The model under review builds one solid part; all positions refer to its coordinate system, in mm. A direction names the side the tool comes from. Give positions to 0.01 mm unless a question says otherwise; leave off trailing zeros. Loops run counter-clockwise (first coordinate to the right, second up) from the corner with the lowest first, then second, coordinate; pieces in that order, holes last. Notation, with made-up numbers: M -2.5,15 L 46.5,15 A26 ccw 46.5,45 Z; hole C -14.5,67 d2. An arc over 180 degrees is marked long. Return JSON: item names as keys, results as strings. Group by question number.
```python
from build123d import *

# Parameters (mm, degrees)
SKETCH1_W            = 58.42
SKETCH1_H            = 27.94
BOSS_EXTRUDE1_DEPTH  = 27.686
SKETCH2_W            = 0.889
SKETCH2_H            = 8.636
SKETCH2_W_2          = 0.254
SKETCH2_H_2          = 1.905
BOSS_EXTRUDE3_DEPTH  = 27.686
CUT_EXTRUDE1_DEPTH   = 27.305
CUT_EXTRUDE3_DEPTH   = 50.528860243
SKETCH6_W            = 0.508
SKETCH6_H            = 1.778
SKETCH6_W_2          = 0.8128
SKETCH6_H_2          = 1.27
SKETCH6_H_3          = 8.636
BOSS_EXTRUDE4_DEPTH  = 27.686
SKETCH7_W            = 1.3462
SKETCH7_H            = 6.223
CUT_EXTRUDE4_DEPTH   = 25.4
SKETCH8_R            = 1.651
CUT_EXTRUDE5_DEPTH   = 44.216030588
SKETCH9_R            = 2.54
CUT_EXTRUDE6_DEPTH   = 25.4
BOSS_EXTRUDE5_DEPTH  = 1.016
MIRROR3_COPY_1_DEPTH = 1.016


with BuildPart() as part:
    # Sketch1 → Boss-Extrude1 (new body)
    with BuildSketch(Plane.XY):
        Rectangle(SKETCH1_W, SKETCH1_H)
    extrude(amount=BOSS_EXTRUDE1_DEPTH)

    # Sketch2 → Boss-Extrude3 (add)
    with BuildSketch(Plane.XY.offset(27.686)):
        with Locations((-29.6545, 0)):
            Rectangle(SKETCH2_W, SKETCH2_H)
        with Locations((-29.337, 13.0175)):
            Rectangle(SKETCH2_W_2, SKETCH2_H_2)
        with Locations((-29.337, -13.0175)):
            Rectangle(SKETCH2_W_2, SKETCH2_H_2)
        with Locations((29.337, -13.0175)):
            Rectangle(SKETCH2_W_2, SKETCH2_H_2)
        with Locations((29.337, 13.0175)):
            Rectangle(SKETCH2_W_2, SKETCH2_H_2)
        with Locations((29.6545, 0)):
            Rectangle(SKETCH2_W, SKETCH2_H)
    extrude(amount=-BOSS_EXTRUDE3_DEPTH)

    # Sketch4 → Cut-Extrude1 (cut, symmetric)
    with BuildSketch(Plane(origin=(0, 0, 0), x_dir=(0, 0, -1), z_dir=(1, 0, 0))):
        with BuildLine():
            Line((-15.5575, 13.0175), (-27.686, 13.0175))
            Line((-27.686, 13.0175), (-27.686, -13.0175))
            Line((-27.686, -13.0175), (-15.5575, -13.0175))
            ThreePointArc((-15.5575, -13.0175), (-2.54, 0), (-15.5575, 13.0175))
        make_face()
    extrude(amount=CUT_EXTRUDE1_DEPTH, both=True, mode=Mode.SUBTRACT)

    # Sketch5 → Cut-Extrude3 (cut, through all)
    with BuildSketch(Plane.XZ.offset(13.97)):
        with BuildLine():
            Line((-27.305, 27.686), (-27.305, 18.669))
            Line((-27.305, 18.669), (-23.037688998, 18.669))
            ThreePointArc((-23.037688998, 18.669), (-21.720466793, 18.382866674), (-20.640662648, 17.576039787))
            Line((-20.640662648, 17.576039787), (-15.589726503, 11.760960213))
            ThreePointArc((-15.589726503, 11.760960213), (-14.509922358, 10.954133326), (-13.192700152, 10.668))
            Line((-13.192700152, 10.668), (-10.541, 10.668))
            ThreePointArc((-10.541, 10.668), (-8.29593597, 9.73806403), (-7.366, 7.493))
            Line((-7.366, 7.493), (-7.366, 5.588))
            Line((-7.366, 5.588), (7.366, 5.588))
            Line((7.366, 5.588), (7.366, 7.493))
            ThreePointArc((7.366, 7.493), (8.29593597, 9.73806403), (10.541, 10.668))
            Line((10.541, 10.668), (13.192700152, 10.668))
            ThreePointArc((13.192700152, 10.668), (14.509922358, 10.954133326), (15.589726503, 11.760960213))
            Line((15.589726503, 11.760960213), (20.640662648, 17.576039787))
            ThreePointArc((20.640662648, 17.576039787), (21.720466793, 18.382866674), (23.037688998, 18.669))
            Line((23.037688998, 18.669), (27.305, 18.669))
            Line((27.305, 18.669), (27.305, 27.686))
            Line((27.305, 27.686), (-27.305, 27.686))
        make_face()
    extrude(amount=-CUT_EXTRUDE3_DEPTH, mode=Mode.SUBTRACT)

    # Sketch6 → Boss-Extrude4 (add)
    with BuildSketch(Plane.XY.offset(27.686)):
        with Locations((-27.051, 13.081)):
            Rectangle(SKETCH6_W, SKETCH6_H)
        with Locations((-26.8986, 7.747)):
            Rectangle(SKETCH6_W_2, SKETCH6_H_2)
        with Locations((-26.8986, 0)):
            Rectangle(SKETCH6_W_2, SKETCH6_H_3)
        with Locations((-26.8986, -7.747)):
            Rectangle(SKETCH6_W_2, SKETCH6_H_2)
        with Locations((-27.051, -13.081)):
            Rectangle(SKETCH6_W, SKETCH6_H)
        with Locations((27.051, -13.081)):
            Rectangle(SKETCH6_W, SKETCH6_H)
        with Locations((26.8986, -7.747)):
            Rectangle(SKETCH6_W_2, SKETCH6_H_2)
        with Locations((26.8986, 0)):
            Rectangle(SKETCH6_W_2, SKETCH6_H_3)
        with Locations((26.8986, 7.747)):
            Rectangle(SKETCH6_W_2, SKETCH6_H_2)
        with Locations((27.051, 13.081)):
            Rectangle(SKETCH6_W, SKETCH6_H)
    extrude(amount=-BOSS_EXTRUDE4_DEPTH)

    # Sketch7 → Cut-Extrude4 (cut)
    with BuildSketch(Plane.XY.offset(27.686)):
        with Locations((-27.1653, 0)):
            Rectangle(SKETCH7_W, SKETCH7_H)
        with Locations((27.1653, 0)):
            Rectangle(SKETCH7_W, SKETCH7_H)
    extrude(amount=-CUT_EXTRUDE4_DEPTH, mode=Mode.SUBTRACT)

    # Sketch8 → Cut-Extrude5 (cut, through all)
    with BuildSketch(Plane.XY.offset(27.686)):
        with Locations((-17.272, 0)):
            Circle(SKETCH8_R)
        with Locations((17.272, 0)):
            Circle(SKETCH8_R)
    extrude(amount=-CUT_EXTRUDE5_DEPTH, mode=Mode.SUBTRACT)

    # Sketch9 → Cut-Extrude6 (cut)
    with BuildSketch(Plane.XY.offset(27.686)):
        with Locations((-17.272, 0)):
            Circle(SKETCH9_R)
        with Locations((17.272, 0)):
            Circle(SKETCH9_R)
    extrude(amount=-CUT_EXTRUDE6_DEPTH, mode=Mode.SUBTRACT)

    # Sketch10 → Boss-Extrude5 (add)
    with BuildSketch(Plane(origin=(0, 0, 0), x_dir=(-1, 0, 0), z_dir=(0, 0, -1))):
        Polygon((-28.963662415, 10.647390084), (-28.963662415, 13.695390084), (-24.137662415, 13.695390084), (-24.137662415, 12.425390084), (-27.693662415, 12.425390084), (-27.693662415, 10.647390084), align=None)
    boss_extrude5 = extrude(amount=BOSS_EXTRUDE5_DEPTH)

    # Mirror2: Boss-Extrude5 across plane
    add(boss_extrude5.mirror(Plane.ZX))

    # Mirror3: Boss-Extrude5 across plane
    add(boss_extrude5.mirror(Plane(origin=(0, 0, 0), x_dir=(0, 0, 1), z_dir=(1, 0, 0))))

    # Mirror3 copy 1 sketch → Mirror3 copy 1 (add)
    with BuildSketch(Plane(origin=(0, 0, 0), x_dir=(1, 0, 0), z_dir=(0, 0, -1))):
        Polygon((-28.963662415, 10.647390084), (-28.963662415, 13.695390084), (-24.137662415, 13.695390084), (-24.137662415, 12.425390084), (-27.693662415, 12.425390084), (-27.693662415, 10.647390084), align=None)
    extrude(amount=MIRROR3_COPY_1_DEPTH)


solid = part.part
```
(1) For pin 1 (6 mm diameter, centred on y = 8.5, z = 23, fed in from -X); pin 2 (0.5 mm diameter, centred on y = 12.5, z = 21.5, fed in from +X); pin 3 (12 mm diameter, centred on x = 18.5, y = 5.5, fed in from +Z), all flat-tipped, find the tip position at first contact; note any pin that passes through.
(2) For probe 1 along X at (y, z) = (0, 2.4); probe 2 along Y at (x, z) = (27, 7.5); probe 3 along X at (y, z) = (5, 11) (3 decimals), list the stretches that pass through material, from the lowest coordinate up.
(3) Mouldability with a two-part tool opening along X and no side actions: class faces 1 (the flat face through (28, 0, 27.686)), 2 (the flat face through (-29.21, 8, 14)), 3 (the cylindrical face through (21.703, 13.487, 18.375)) as released by +X, released by -X, zero draft, split by the parting line, or undercut.
(4) Add section A-A (y = 0). Write out the cut boundary in (x, z), and give its area (3 significant figures).
(5) For faces 4 (the cylindrical face through (21.703, -13.5, 18.375)), 5 (the flat face through (-30.099, 0, 14)), 6 (the flat face through (-26.492, 8, 16)), 7 (the flat face through (-29.21, -8, 14)), 8 (the flat face through (29.464, -13, 14)), list the 3-axis set-ups (+Z, -Z, +X, -X, +Y, -Y) from which the entire face can be reached by the end or side of a thin tool; tool diameter is ignored.
Verdict:
{
 "1": {"pin 1": "stops at x = -29.21", "pin 2": "stops at x = 29.46", "pin 3": "stops at z = 9.46"},
 "2": {"probe 1": "x = -30.1 to -27.84, -26.49 to -19.81, -14.73 to 14.73, 19.81 to 26.49, 27.84 to 30.1", "probe 2": "y = -13.97 to -10.22, -8.38 to -7.11, -4.32 to -3.11, 3.11 to 4.32, 7.11 to 8.38, 10.22 to 13.97", "probe 3": "x = -29.21 to -27.305, 27.305 to 29.21"},
 "3": {"face 1": "zero draft", "face 2": "released by -X", "face 3": "undercut"},
 "4": {"outline": "M -30.1,0 L -18.92,0 L -18.92,2.29 L -19.81,2.29 L -19.81,2.54 L -26.49,2.54 L -26.49,2.29 L -27.84,2.29 L -27.84,27.69 L -30.1,27.69 Z; M -15.62,0 L 15.62,0 L 15.62,2.29 L 14.73,2.29 L 14.73,2.54 L -14.73,2.54 L -14.73,2.29 L -15.62,2.29 Z; M 18.92,0 L 30.1,0 L 30.1,27.69 L 27.84,27.69 L 27.84,2.29 L 26.49,2.29 L 26.49,2.54 L 19.81,2.54 L 19.81,2.29 L 18.92,2.29 Z", "area": "248 mm²"},
 "5": {"face 4": "+Z, +Y, -Y", "face 5": "+Z, -Z, -X, +Y, -Y", "face 6": "+Z", "face 7": "+Z, -Z, -X", "face 8": "+Z, -Z, +X, -Y"}
}
